The listing builds one solid part. Answer for the finished solid, in the listing's coordinates (mm). A direction names the side the tool comes from. Coordinates: 2 decimals unless noted, no trailing zeros. Order: outer loops, then holes, each group sorted by start corner. A loop starts at its lowest first (then second) coordinate and runs counter-clockwise, first axis right, second up. Notation, with made-up numbers: (75, 20.25) -> (113, 20.25) arc R17 cw to (113, 42.25) -> close; hole circle Ø6 at (52, -1). An arc over 180 degrees is marked (long way). Answer in a Markdown table with one row per item. Add a question column.
Autodesk Inventor part; units mm, degrees
ref_plane "YZ Plane" through (0, 0, 0) normal (1, 0, 0) x (0, 1, 0)
ref_plane "XZ Plane" through (0, 0, 0) normal (0, 1, 0) x (-1, 0, 0)
ref_plane "XY Plane" through (0, 0, 0) normal (0, 0, 1) x (1, 0, 0)
sketch "スケッチ2" plane through (0, 0, 0) normal (0, 1, 0) x (-1, 0, 0)
  line L0 (0, 0) -> (-77.8, 0)
  line L1 (-77.8, 0) -> (-77.8, -40)
  line L2 (-77.8, -40) -> (0, -40)
  line L3 (0, -40) -> (0, 0)
  dimension "d0" = 77.8
  dimension "d1" = 40
extrude "押し出し1" add sketch "スケッチ2" along normal blind 5
sketch "スケッチ4" plane through (0, 0, -40) normal (-1, 0, 0) x (0, 0, 1)
  line L0 (0, 0) -> (0, 5) construction
  line L1 (0, 2.5) -> (40, 2.5) construction
  line L2 (40, 0) -> (40, 5) construction
  point P0 (4, 2.5)
  point P1 (36, 2.5)
  dimension "d4" = 4
  dimension "d5" = 4
hole "穴1" at (0, 2.5, -36) at (0, 2.5, -4) direction (1, 0, 0) diameter 2.459 depth 12
sketch "スケッチ5" plane through (77.8, 0, 0) normal (1, 0, 0) x (0, 0, -1)
  line L0 (0, 0) -> (0, 5) construction
  line L1 (0, 2.5) -> (39.9198, 2.5) construction
  circle A0 centre (4, 2.5) radius 1.2295 construction
  circle A1 centre (36, 2.5) radius 1.2295
  point P0 (4, 2.5)
  point P1 (36, 2.5)
hole "穴2" at (77.8, 2.5, -4) at (77.8, 2.5, -36) direction (-1, 0, 0) diameter 2.459 depth 13
sketch "スケッチ6" plane through (0, 5, 0) normal (0, 1, 0) x (1, 0, 0)
  line L0 (77.8, 0) -> (77.8, 40) construction
  line L1 (0, 40) -> (0, 0) construction
  line L2 (0, 0) -> (77.8, 0) construction
  point P0 (57.3, 12.5)
  dimension "d20" = 20.5
  dimension "d21" = 12.5
hole "穴3" at (57.3, 5, -12.5) direction (0, -1, 0) diameter 8.1 end through all
sketch "スケッチ7" plane through (0, 5, 0) normal (0, 1, 0) x (1, 0, 0)
  line L0 (77.8, 0) -> (77.8, 40) construction
  line L1 (77.8, 28.3) -> (0, 28.3) construction
  line L2 (0, 40) -> (0, 0) construction
  circle A0 centre (57.3, 12.5) radius 4.05 construction
  point P0 (67.8, 28.3)
  point P1 (46.8, 28.3)
  dimension "d29" = 15.8
  dimension "d30" = 10.5
  dimension "d31" = 10.5
hole "穴4" [suppressed]
sketch "スケッチ11" plane through (0, 5, 0) normal (0, 1, 0) x (1, 0, 0)
  circle A0 centre (57.3, 12.5) radius 4.05
  line L0 (55.8, 7.05) -> (58.8, 7.05)
  line L1 (58.8, 7.05) -> (58.8, 8.45)
  line L2 (58.8, 8.45) -> (55.8, 8.45)
  line L3 (55.8, 8.45) -> (55.8, 7.05)
  line L4 (55.8, 8.45) -> (55.8, 8.738)
  line L5 (58.8, 8.45) -> (58.8, 8.738)
  point P0 (0, 0)
  point P1 (57.3, 8.45)
  dimension "d68" = 1.4
  dimension "d69" = 3
extrude "押し出し3" cut sketch "スケッチ11" against normal through all contours A0 L2 L4 | L5 L2 A0 | L2 L1 L0 L3
sketch "スケッチ8" plane through (0, 5, 0) normal (0, 1, 0) x (1, 0, 0)
  arc A0 (58.8, 8.738) -> (55.8, 8.738) centre (57.3, 12.5) ccw construction
  circle A1 centre (57.3, 12.5) radius 7 construction
  point P0 (0, 0)
  point P1 (57.3, 19.5)
  point P2 (50.3, 12.5)
  point P3 (64.3, 12.5)
  dimension "d39" = 14
hole "穴5" at (57.3, 5, -19.5) at (50.3, 5, -12.5) at (64.3, 5, -12.5) direction (0, -1, 0) diameter 2.459 end through all
sketch "スケッチ9" plane through (0, 5, 0) normal (0, 1, 0) x (1, 0, 0)
  circle A0 centre (57.3, 12.5) radius 4.05
  line L0 (57.3, 12.5) -> (45.9478, 12.5) construction
  line L1 (51.85, 14) -> (53.25, 14)
  line L2 (53.25, 14) -> (53.25, 11)
  line L3 (53.25, 11) -> (51.85, 11)
  line L4 (51.85, 11) -> (51.85, 14)
  line L5 (51.85, 14) -> (53.25, 11) construction
  line L6 (53.25, 14) -> (51.85, 11) construction
  line L7 (53.25, 11) -> (53.538, 11)
  line L8 (53.25, 14) -> (53.538, 14)
  point P0 (0, 0)
  point P1 (52.55, 12.5)
  point P2 (53.25, 12.5)
  dimension "d56" = 1.4
  dimension "d57" = 0
  dimension "d58" = 3
extrude "押し出し2" [suppressed]
sketch "スケッチ12" plane through (0, 5, 0) normal (0, 1, 0) x (1, 0, 0)
  arc A0 (58.8, 8.738) -> (55.8, 8.738) centre (57.3, 12.5) ccw
  point P0 (0, 0)
  point P1 (50.3, 12.5)
  point P2 (57.3, 5.5)
  point P3 (64.3, 12.5)
  point P4 (57.3, 19.5)
  dimension "d74" = 360
  dimension "d76" = 14
hole "穴7" [suppressed]
sketch "スケッチ13" plane through (0, 0, 0) normal (0, 0, 1) x (1, 0, 0)
  line L0 (58.8, 5) -> (55.8, 5)
  line L1 (77.8, 0) -> (77.8, 5)
  point P0 (0, 0)
  point P1 (57.3, 2.5)
  point P2 (57.3, 5)
  point P3 (77.8, 2.5)
hole "穴8" at (57.3, 2.5, 0) direction (0, 0, -1) diameter 1.567 depth 7.05
properties part number "shoulder1_verticval_cover" material "アルミニウム 5052"
Q1. A cutting plane is placed at C-C (x = 9). Determine the outline of the cut face in (y, z), then the cut area to 3 significant figures.
Q2. A cutting plane is placed at B-B (z = -12.5). Determine the outline of the cut face in (x, y).
Q3. Straight lines are drawn through the part: line 1 (Z direction, x = 69, y = 2.4); line 2 (X direction, y = 1.5, z = -12.5); line 3 (Z direction, x = 57.3, y = 2.6). For each, find the intervals that lie inside material, in ascending order.
Q4. A cutting plane is placed at A-A (x = 50.3). Determine the outline of the cut face in (y, z).
Q5. A cutting plane is placed at D-D (z = -36). Determine the outline of the cut face in (x, y), then the cut area to 3 significant figures.
Q6. For faces 1 (the face through (12, 2, -36)), 2 (the face through (58.8, 3, -8)), 3 (the face through (71.21, 2.45, -2.77)), 4 (the face through (56.523, 2.602, -3.574)), determine the directions among +Z, -Z, +X, -X, +Y, -Y from which every point of the face is accessible in a straight line to the end or side of a thin tool.
Q7. Determine the mould class of faces 5 (the face through (38, 2, 0)), 6 (the face through (64.8, 2, -4)), 7 (the face through (71.209, 2.131, -37.173)), 8 (the face through (39, 0, -20)) for opening direction Y: +Y half, -Y half, draft (parallel to the pull), parting line (faces both ways), or undercut.
Q8. Given pin 1 (1.5 mm diameter, centred on y = 2.5, z = -36, fed in from -X); pin 2 (1.2 mm diameter, centred on y = 2, z = -36, fed in from +X), each flat-ended and moving along its own axis, determine where each tip first touches the part or whether it passes through.
Returned:
| question | item | result |
|---|---|---|
| 1 | outline | (0, -40) -> (5, -40) -> (5, 0) -> (0, 0) -> close; hole circle Ø2.46 at (2.5, -36); hole circle Ø2.46 at (2.5, -4) |
| 1 | area | 191 mm² |
| 2 | outline | (0, 0) -> (49.07, 0) -> (49.07, 5) -> (0, 5) -> close; (51.53, 0) -> (53.25, 0) -> (53.25, 5) -> (51.53, 5) -> close; (61.35, 0) -> (63.07, 0) -> (63.07, 5) -> (61.35, 5) -> close; (65.53, 0) -> (77.8, 0) -> (77.8, 5) -> (65.53, 5) -> close |
| 3 | line 1 | z = -40 to -37.23, -34.77 to -5.23, -2.77 to 0 |
| 3 | line 2 | x = 0 to 49.07, 51.53 to 53.25, 61.35 to 63.07, 65.53 to 77.8 |
| 3 | line 3 | z = -40 to -20.73, -18.27 to -16.55 |
| 4 | outline | (0, -40) -> (5, -40) -> (5, -13.73) -> (0, -13.73) -> close; (0, -11.27) -> (5, -11.27) -> (5, 0) -> (0, 0) -> close |
| 5 | outline | (0, 0) -> (77.8, 0) -> (77.8, 1.27) -> (64.8, 1.27) -> (64.8, 3.73) -> (77.8, 3.73) -> (77.8, 5) -> (0, 5) -> (0, 3.73) -> (12, 3.73) -> (12, 1.27) -> (0, 1.27) -> close |
| 5 | area | 328 mm² |
| 6 | face 1 | -X |
| 6 | face 2 | +Y, -Y |
| 6 | face 3 | +X |
| 6 | face 4 | +Z |
| 7 | face 5 | draft |
| 7 | face 6 | undercut |
| 7 | face 7 | undercut |
| 7 | face 8 | -Y half |
| 8 | pin 1 | stops at x = 12 |
| 8 | pin 2 | stops at x = 64.8 |
